For this review, take the finished solid that the model builds, in its own axes (mm). Coordinates: 2 decimals unless noted, no trailing zeros. Write each loop counter-clockwise with the first axis right and the second up, starting at its lowest first coordinate (ties: lowest second). Pieces come first, ordered by that corner, then holes.
1) To check wall thickness, follow line 1 along Y through (x, z) = (1.75, -10.75); line 2 along Y through (x, z) = (3, -11.5); line 3 along Z through (x, y) = (-3.75, 8.25). State the ranges of each line that lie inside material, in increasing order.
2) Insertion check: P1, Ø1.5, axis at y = 8, z = 3.5, coming from the -X side. The pin has a flat end and moves straight along its axis. Give the tip position at first contact, or say it passes through.
3) We need section A-A on y = 8.5. Write out the cut boundary in (x, z), then the cut area to 3 significant figures.
Autodesk Inventor part; units mm, degrees
ref_plane "YZ Plane" through (0, 0, 0) normal (1, 0, 0) x (0, 1, 0)
ref_plane "XZ Plane" through (0, 0, 0) normal (0, 1, 0) x (-1, 0, 0)
ref_plane "XY Plane" through (0, 0, 0) normal (0, 0, 1) x (1, 0, 0)
sketch "Эскиз1" plane through (0, 0, 0) normal (0, 1, 0) x (-1, 0, 0)
  line L0 (-12.5, 12.5) -> (12.5, 12.5)
  line L1 (12.5, 12.5) -> (12.5, -12.5)
  line L2 (12.5, -12.5) -> (-12.5, -12.5)
  line L3 (-12.5, -12.5) -> (-12.5, 12.5)
  line L4 (-12.5, 12.5) -> (12.5, -12.5) construction
  line L5 (12.5, 12.5) -> (-12.5, -12.5) construction
  point P0 (0, 0)
  dimension "d0" = 25
extrude "Выдавливание1" add sketch "Эскиз1" along normal blind 9
fillet "Сопряжение1" radius 2 4 edges at (0, 9, 12.5) (12.5, 9, 0) (0, 9, -12.5) (-12.5, 9, 0)
properties part number "Антена GPS" material "Сталь нержавеющая, 440C"
Result:
1. line 1: y = 0 to 8.98
1. line 2: y = 0 to 8.73
1. line 3: z = -12.06 to 12.06
2. P1: stops at x = -12.48
3. outline: (-11.82, -11.82) - (11.82, -11.82) - (11.82, 11.82) - (-11.82, 11.82) - close
3. area: 559 mm2
